The listing builds one solid part. Answer for the finished solid, in the listing's coordinates (mm). Face numbers are marked on the shaded views. A direction names the side the tool comes from. Give positions to 0.01 mm unless a question says otherwise; leave off trailing zeros. Loops run counter-clockwise (first coordinate to the right, second up) from the corner with the lowest first, then second, coordinate; pieces in that order, holes last. Notation, with made-up numbers: (62.5, -3.5) - (103.5, -3.5) arc R20 cw to (103.5, 5.5) - close; hole circle Ø3 at (6.25, 88). An arc over 180 degrees is marked (long way). Answer as CSV lines item,"result". Start each with the question number.
1) Flat-ended cylindrical pins translate along their axes: pin 1 (5 mm diameter, centred on x = -31, z = 5, fed in from +Y); pin 2 (4 mm diameter, centred on x = -24, y = -103.5, fed in from +Z); pin 3 (2 mm diameter, centred on x = 46, y = -12, fed in from +Z); pin 4 (2 mm diameter, centred on x = 22.5, z = 10.5, fed in from -Y). Find the tip coordinate at first contact, or state that the pin passes through.
2) A cutting plane is placed at B-B (y = -99). Determine the outline of the cut face in (x, z).
3) A cutting plane is placed at D-D (y = -136). Determine the outline of the cut face in (x, z).
4) For a pull along X with two mould halves and no side action, classify the marked faces 3, 4 and 5 as pulls with the +X half, pulls with the -X half, needs draft (parallel to the pull), parting line crosses it, or undercut.
5) A cutting plane is placed at C-C (x = -3.5). Determine the outline of the cut face in (y, z), and give its area (3 significant figures).
6) A cutting plane is placed at A-A (z = 7). Determine the outline of the cut face in (x, y).
7) Find the intervals of material crossed by line 1 along Y through (x, z) = (0, 30.5); line 2 along Y through (x, z) = (39.5, 2); line 3 along Y through (x, z) = (8, 6), in increasing order.
8) For the marked faces 1 and 2, determine the directions among +Z, -Z, +X, -X, +Y, -Y from which every point of the face is accessible in a straight line to the end or side of a thin tool.
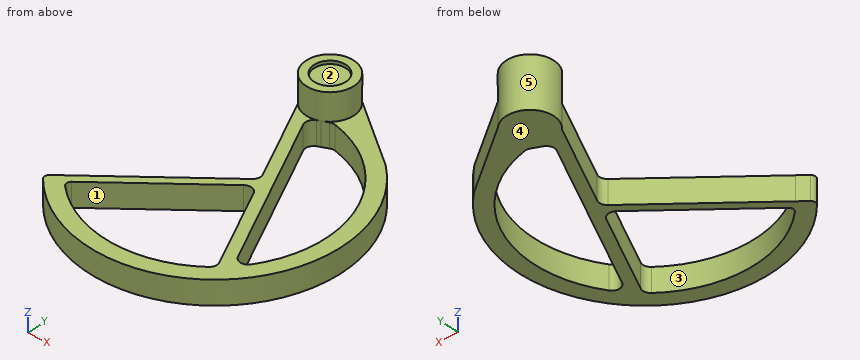
```python
from build123d import *

# Parameters (mm, degrees)
EXTRUDE_1_DEPTH     = 15
CUT_EXTRUDE_START   = -15
CUT_EXTRUDE_1_DEPTH = 15
SKETCH_9_R          = 15
EXTRUDE_2_DEPTH     = 17
SKETCH_10_R         = 10
CUT_EXTRUDE_4_DEPTH = 2


with BuildPart() as part:
    # ｽｹｯﾁ4 → ﾎﾞｽ - 押し出し1 (new body)
    with BuildSketch(Plane.XY):
        with BuildLine():
            Line((-53.623111018, -124.995132678), (-58.940636287, -129.45706617))
            ThreePointArc((-58.940636287, -129.45706617), (-60.005384698, -131.552012131), (-59.233530865, -133.771635843))
            ThreePointArc((-59.233530865, -133.771635843), (57.362306223, -135.763481103), (52.076178918, -19.270504783))
            Line((52.076178918, -19.270504783), (10.606601718, 10.606601718))
            ThreePointArc((10.606601718, 10.606601718), (-10.606601718, 10.606601718), (-10.606601718, -10.606601718))
            Line((-10.606601718, -10.606601718), (14.536280154, -62.889638219))
            ThreePointArc((14.536280154, -62.889638219), (14.918089499, -66.109676181), (13.244185189, -68.886809092))
            Line((13.244185189, -68.886809092), (-53.623111018, -124.995132678))
        make_face()
        with BuildLine():
            Line((21.232400696, -76.813798404), (45.844843506, -127.993820346))
            ThreePointArc((45.844843506, -127.993820346), (46.221944165, -131.235480845), (44.518718993, -134.019289696))
            ThreePointArc((44.518718993, -134.019289696), (-2.231208213, -149.964431749), (-47.870174388, -131.072951785))
            ThreePointArc((-47.870174388, -131.072951785), (-48.817477846, -128.802229421), (-47.747678417, -126.586582094))
            Line((-47.747678417, -126.586582094), (13.511229465, -75.151532228))
            ThreePointArc((13.511229465, -75.151532228), (17.77869109, -74.092739753), (21.232400696, -76.813798404))
        make_face(mode=Mode.SUBTRACT)
    extrude(amount=EXTRUDE_1_DEPTH)

    # ｽｹｯﾁ6 → ｶｯﾄ - 押し出し1 (cut)
    with BuildSketch(Plane.XY.offset(15).offset(CUT_EXTRUDE_START)):
        with BuildLine():
            Line((49.189589797, -118.797265215), (2.201751786, -21.089020696))
            ThreePointArc((2.201751786, -21.089020696), (1.989274209, -17.268089629), (4.540836142, -14.416039025))
            Line((4.540836142, -14.416039025), (6.483415605, -13.48185369))
            Line((6.483415605, -13.48185369), (10.219658847, -11.685096486))
            ThreePointArc((10.219658847, -11.685096486), (11.747077013, -11.232198087), (13.339423466, -11.282754846))
            ThreePointArc((13.339423466, -11.282754846), (64.738421392, -53.37413296), (57.826055334, -119.448033215))
            ThreePointArc((57.826055334, -119.448033215), (53.319931874, -121.616182211), (49.189589797, -118.797265215))
        make_face()
    extrude(amount=CUT_EXTRUDE_1_DEPTH, mode=Mode.SUBTRACT)

    # ｽｹｯﾁ9 → ﾎﾞｽ - 押し出し2 (add)
    with BuildSketch(Plane.XY.offset(15)):
        with Locations(Location((0, 0, 0), (0, 0, 225))):
            Circle(SKETCH_9_R)
    extrude(amount=EXTRUDE_2_DEPTH)

    # ｽｹｯﾁ10 → ｶｯﾄ - 押し出し4 (cut)
    with BuildSketch(Plane.XY.offset(32)):
        Circle(SKETCH_10_R)
    extrude(amount=-CUT_EXTRUDE_4_DEPTH, mode=Mode.SUBTRACT)


solid = part.part
```
Ans:
1,pin 1,"y = -103.91"
1,pin 2,"z = 15"
1,pin 3,"through"
1,pin 4,"y = -157.06"
2,outline,"(-22.64, 0) - (-14.89, 0) - (-14.89, 15) - (-22.64, 15) - close; (31.9, 0) - (39.67, 0) - (39.67, 15) - (31.9, 15) - close; (67.37, 0) - (77.71, 0) - (77.71, 15) - (67.37, 15) - close"
3,outline,"(-57.13, 0) - (-42, 0) - (-42, 15) - (-57.13, 15) - close; (42, 0) - (57.13, 0) - (57.13, 15) - (42, 15) - close"
4,face 3,"undercut"
4,face 4,"needs draft"
4,face 5,"parting line crosses it"
5,outline,"(-159.92, 0) - (-149.91, 0) - (-149.91, 15) - (-159.92, 15) - close; (-89.43, 0) - (-82.94, 0) - (-82.94, 15) - (-89.43, 15) - close; (-25.38, 0) - (14.59, 0) - (14.59, 32) - (9.37, 32) - (9.37, 30) - (-9.37, 30) - (-9.37, 32) - (-14.59, 32) - (-14.59, 15) - (-25.38, 15) - close"
5,area,"1,310 mm2"
6,outline,"(-59.23, -133.77) arc R80 ccw (long way) to (52.08, -19.27) - (10.61, 10.61) arc R15 ccw to (-10.61, -10.61) - (14.54, -62.89) arc R5 cw to (13.24, -68.89) - (-58.94, -129.46) arc R3 ccw to start; hole (-47.87, -131.07) arc R70 ccw to (44.52, -134.02) arc R5 ccw to (45.84, -127.99) - (21.23, -76.81) arc R5 ccw to (13.51, -75.15) - (-47.75, -126.59) arc R3 ccw to start; hole (2.2, -21.09) - (49.19, -118.8) arc R5 ccw to (57.83, -119.45) arc R70 ccw to (13.34, -11.28) arc R5 ccw to (10.22, -11.69) - (4.54, -14.42) arc R5 ccw to start"
7,line 1,"-15 to -10, 10 to 15"
7,line 2,"-149.57 to -137.79, -114.8 to -98.65, -22.21 to -10.21"
7,line 3,"-159.6 to -149.54, -79.78 to -73.29, -49.3 to -33.15, -12.75 to 12.69"
8,face 1,"+Z, -Z"
8,face 2,"+Z"
